```python
from build123d import *

# Parameters (mm, degrees)
BOSS_EXTRUDE1_DEPTH = 4
BOSS_EXTRUDE2_DEPTH = 8
BOSS_EXTRUDE3_DEPTH = 4
SKETCH4_R           = 2.6
CUT_EXTRUDE1_DEPTH  = 12
SKETCH5_W           = 20
SKETCH5_H           = 20
CUT_EXTRUDE2_DEPTH  = 12


with BuildPart() as part:
    # Sketch1 → Boss-Extrude1 (new body)
    with BuildSketch(Plane(origin=(0, 0, 0), x_dir=(1, 0, 0), z_dir=(0, 1, 0))):
        with BuildLine():
            Line((21.403642989, 12.918361615), (25.455844123, 16.970562748))
            ThreePointArc((25.455844123, 16.970562748), (25.455844123, 25.455844123), (16.970562748, 25.455844123))
            Line((16.970562748, 25.455844123), (12.918361615, 21.403642989))
            ThreePointArc((12.918361615, 21.403642989), (0, 25), (-12.918361615, 21.403642989))
            Line((-12.918361615, 21.403642989), (-16.970562748, 25.455844123))
            ThreePointArc((-16.970562748, 25.455844123), (-25.455844123, 25.455844123), (-25.455844123, 16.970562748))
            Line((-25.455844123, 16.970562748), (-21.403642989, 12.918361615))
            ThreePointArc((-21.403642989, 12.918361615), (-25, 0), (-21.403642989, -12.918361615))
            Line((-21.403642989, -12.918361615), (-25.455844123, -16.970562748))
            ThreePointArc((-25.455844123, -16.970562748), (-25.455844123, -25.455844123), (-16.970562748, -25.455844123))
            Line((-16.970562748, -25.455844123), (-12.918361615, -21.403642989))
            ThreePointArc((-12.918361615, -21.403642989), (0, -25), (12.918361615, -21.403642989))
            Line((12.918361615, -21.403642989), (16.970562748, -25.455844123))
            ThreePointArc((16.970562748, -25.455844123), (25.455844123, -25.455844123), (25.455844123, -16.970562748))
            Line((25.455844123, -16.970562748), (21.403642989, -12.918361615))
            ThreePointArc((21.403642989, -12.918361615), (25, 0), (21.403642989, 12.918361615))
        make_face()
    extrude(amount=BOSS_EXTRUDE1_DEPTH)

    # Sketch2 → Boss-Extrude2 (add)
    with BuildSketch(Plane(origin=(0, 4, 0), x_dir=(1, 0, 0), z_dir=(0, 1, 0))):
        with BuildLine():
            Line((-1, 25), (-1, 22.477766793))
            ThreePointArc((-1, 22.477766793), (-4.389532245, 22.067668809), (-7.677989416, 21.149432109))
            Line((-7.677989416, 21.149432109), (-8.643206277, 23.479671745))
            ThreePointArc((-8.643206277, 23.479671745), (-9.574736419, 23.115458518), (-10.490965342, 22.71430488))
            Line((-10.490965342, 22.71430488), (-9.525748481, 20.384065244))
            ThreePointArc((-9.525748481, 20.384065244), (-10.316353506, 19.995570768), (-11.091145538, 19.576426912))
            Line((-11.091145538, 19.576426912), (-16.970562748, 25.455844123))
            ThreePointArc((-16.970562748, 25.455844123), (-25.455844123, 25.455844123), (-25.455844123, 16.970562748))
            Line((-25.455844123, 16.970562748), (-19.576426912, 11.091145538))
            ThreePointArc((-19.576426912, 11.091145538), (-19.995570768, 10.316353506), (-20.384065244, 9.525748481))
            Line((-20.384065244, 9.525748481), (-22.71430488, 10.490965342))
            ThreePointArc((-22.71430488, 10.490965342), (-23.115458518, 9.574736419), (-23.479671745, 8.643206277))
            Line((-23.479671745, 8.643206277), (-21.149432109, 7.677989416))
            ThreePointArc((-21.149432109, 7.677989416), (-22.067668809, 4.389532245), (-22.477766793, 1))
            Line((-22.477766793, 1), (-25, 1))
            ThreePointArc((-25, 1), (-25.019992006, 0), (-25, -1))
            Line((-25, -1), (-22.477766793, -1))
            ThreePointArc((-22.477766793, -1), (-22.067668809, -4.389532245), (-21.149432109, -7.677989416))
            Line((-21.149432109, -7.677989416), (-23.479671745, -8.643206277))
            ThreePointArc((-23.479671745, -8.643206277), (-23.115458518, -9.574736419), (-22.71430488, -10.490965342))
            Line((-22.71430488, -10.490965342), (-20.384065244, -9.525748481))
            ThreePointArc((-20.384065244, -9.525748481), (-19.995570768, -10.316353506), (-19.576426912, -11.091145538))
            Line((-19.576426912, -11.091145538), (-25.455844123, -16.970562748))
            ThreePointArc((-25.455844123, -16.970562748), (-25.455844123, -25.455844123), (-16.970562748, -25.455844123))
            Line((-16.970562748, -25.455844123), (-11.091145538, -19.576426912))
            ThreePointArc((-11.091145538, -19.576426912), (-10.316353506, -19.995570768), (-9.525748481, -20.384065244))
            Line((-9.525748481, -20.384065244), (-10.490965342, -22.71430488))
            ThreePointArc((-10.490965342, -22.71430488), (-9.574736419, -23.115458518), (-8.643206277, -23.479671745))
            Line((-8.643206277, -23.479671745), (-7.677989416, -21.149432109))
            ThreePointArc((-7.677989416, -21.149432109), (-4.389532245, -22.067668809), (-1, -22.477766793))
            Line((-1, -22.477766793), (-1, -25))
            ThreePointArc((-1, -25), (0, -25.019992006), (1, -25))
            Line((1, -25), (1, -22.477766793))
            ThreePointArc((1, -22.477766793), (4.389532245, -22.067668809), (7.677989416, -21.149432109))
            Line((7.677989416, -21.149432109), (8.643206277, -23.479671745))
            ThreePointArc((8.643206277, -23.479671745), (9.574736419, -23.115458518), (10.490965342, -22.71430488))
            Line((10.490965342, -22.71430488), (9.525748481, -20.384065244))
            ThreePointArc((9.525748481, -20.384065244), (10.316353506, -19.995570768), (11.091145538, -19.576426912))
            Line((11.091145538, -19.576426912), (16.970562748, -25.455844123))
            ThreePointArc((16.970562748, -25.455844123), (25.455844123, -25.455844123), (25.455844123, -16.970562748))
            Line((25.455844123, -16.970562748), (19.576426912, -11.091145538))
            ThreePointArc((19.576426912, -11.091145538), (19.995570768, -10.316353506), (20.384065244, -9.525748481))
            Line((20.384065244, -9.525748481), (22.71430488, -10.490965342))
            ThreePointArc((22.71430488, -10.490965342), (23.115458518, -9.574736419), (23.479671745, -8.643206277))
            Line((23.479671745, -8.643206277), (21.149432109, -7.677989416))
            ThreePointArc((21.149432109, -7.677989416), (22.067668809, -4.389532245), (22.477766793, -1))
            Line((22.477766793, -1), (25, -1))
            ThreePointArc((25, -1), (25.019992006, 0), (25, 1))
            Line((25, 1), (22.477766793, 1))
            ThreePointArc((22.477766793, 1), (22.067668809, 4.389532245), (21.149432109, 7.677989416))
            Line((21.149432109, 7.677989416), (23.479671745, 8.643206277))
            ThreePointArc((23.479671745, 8.643206277), (23.115458518, 9.574736419), (22.71430488, 10.490965342))
            Line((22.71430488, 10.490965342), (20.384065244, 9.525748481))
            ThreePointArc((20.384065244, 9.525748481), (19.995570768, 10.316353506), (19.576426912, 11.091145538))
            Line((19.576426912, 11.091145538), (25.455844123, 16.970562748))
            ThreePointArc((25.455844123, 16.970562748), (25.455844123, 25.455844123), (16.970562748, 25.455844123))
            Line((16.970562748, 25.455844123), (11.091145538, 19.576426912))
            ThreePointArc((11.091145538, 19.576426912), (10.316353506, 19.995570768), (9.525748481, 20.384065244))
            Line((9.525748481, 20.384065244), (10.490965342, 22.71430488))
            ThreePointArc((10.490965342, 22.71430488), (9.574736419, 23.115458518), (8.643206277, 23.479671745))
            Line((8.643206277, 23.479671745), (7.677989416, 21.149432109))
            ThreePointArc((7.677989416, 21.149432109), (4.389532245, 22.067668809), (1, 22.477766793))
            Line((1, 22.477766793), (1, 25))
            ThreePointArc((1, 25), (0, 25.019992006), (-1, 25))
        make_face()
    extrude(amount=BOSS_EXTRUDE2_DEPTH)

    # Sketch3 → Boss-Extrude3 (add)
    with BuildSketch(Plane(origin=(0, 12, 0), x_dir=(1, 0, 0), z_dir=(0, 1, 0))):
        with BuildLine():
            Line((21.403642989, -12.918361615), (25.455844123, -16.970562748))
            ThreePointArc((25.455844123, -16.970562748), (25.455844123, -25.455844123), (16.970562748, -25.455844123))
            Line((16.970562748, -25.455844123), (12.918361615, -21.403642989))
            ThreePointArc((12.918361615, -21.403642989), (0, -25), (-12.918361615, -21.403642989))
            Line((-12.918361615, -21.403642989), (-16.970562748, -25.455844123))
            ThreePointArc((-16.970562748, -25.455844123), (-25.455844123, -25.455844123), (-25.455844123, -16.970562748))
            Line((-25.455844123, -16.970562748), (-21.403642989, -12.918361615))
            ThreePointArc((-21.403642989, -12.918361615), (-25, 0), (-21.403642989, 12.918361615))
            Line((-21.403642989, 12.918361615), (-25.455844123, 16.970562748))
            ThreePointArc((-25.455844123, 16.970562748), (-25.455844123, 25.455844123), (-16.970562748, 25.455844123))
            Line((-16.970562748, 25.455844123), (-12.918361615, 21.403642989))
            ThreePointArc((-12.918361615, 21.403642989), (0, 25), (12.918361615, 21.403642989))
            Line((12.918361615, 21.403642989), (16.970562748, 25.455844123))
            ThreePointArc((16.970562748, 25.455844123), (25.455844123, 25.455844123), (25.455844123, 16.970562748))
            Line((25.455844123, 16.970562748), (21.403642989, 12.918361615))
            ThreePointArc((21.403642989, 12.918361615), (25, 0), (21.403642989, -12.918361615))
        make_face()
    extrude(amount=BOSS_EXTRUDE3_DEPTH)

    # Sketch4 → Cut-Extrude1 (cut)
    with BuildSketch(Plane(origin=(0, 16, 0), x_dir=(1, 0, 0), z_dir=(0, 1, 0))):
        with Locations(Location((-21.213203436, -21.213203436, 0), (0, 0, 270))):
            Circle(SKETCH4_R)
        with Locations(Location((-21.213203436, 21.213203436, 0), (0, 0, 270))):
            Circle(SKETCH4_R)
        with Locations(Location((21.213203436, 21.213203436, 0), (0, 0, 270))):
            Circle(SKETCH4_R)
        with Locations(Location((21.213203436, -21.213203436, 0), (0, 0, 270))):
            Circle(SKETCH4_R)
    extrude(amount=-CUT_EXTRUDE1_DEPTH, mode=Mode.SUBTRACT)

    # Sketch5 → Cut-Extrude2 (cut)
    with BuildSketch(Plane(origin=(0, 16, 0), x_dir=(1, 0, 0), z_dir=(0, 1, 0))):
        Rectangle(SKETCH5_W, SKETCH5_H)
    extrude(amount=-CUT_EXTRUDE2_DEPTH, mode=Mode.SUBTRACT)


solid = part.part
```
Read the model definition and answer for the solid it produces. Units are mm, in the model's axes. A direction names the side the tool comes from. Give positions to 0.01 mm unless a question says otherwise; leave off trailing zeros. Order: outer loops, then holes, each group sorted by start corner. A loop starts at its lowest first (then second) coordinate and runs counter-clockwise, first axis right, second up. Notation, with made-up numbers: (-7, 0) -> (26, 0) arc R23 ccw to (26, 25) -> close; hole circle Ø11 at (67, 35.5). An arc over 180 degrees is marked (long way). Write item = value, one per line.
1. A cutting plane is placed at D-D, the plane y = 9. Count the separate pieces of the cut face and the enclosed holes in it, and give its area (3 significant figures).
Numbers:
separate_pieces = 1
enclosed_holes = 5
area = 1,770 mm²
2. A cutting plane is placed at B-B, the plane z = -3.5. Write down the section's boundary in (x, y).
Numbers:
outline = (-24.75, 0) -> (24.75, 0) -> (24.75, 4) -> (22.23, 4) -> (22.23, 12) -> (24.75, 12) -> (24.75, 16) -> (10, 16) -> (10, 4) -> (-10, 4) -> (-10, 16) -> (-24.75, 16) -> (-24.75, 12) -> (-22.23, 12) -> (-22.23, 4) -> (-24.75, 4) -> close
3. A cutting plane is placed at A-A, the plane y = 1. Write down the section's boundary in (x, z), and give its area (3 significant figures).
Numbers:
outline = (-25.46, -16.97) arc R6 ccw to (-16.97, -25.46) -> (-12.92, -21.4) arc R25 ccw to (12.92, -21.4) -> (16.97, -25.46) arc R6 ccw to (25.46, -16.97) -> (21.4, -12.92) arc R25 ccw to (21.4, 12.92) -> (25.46, 16.97) arc R6 ccw to (16.97, 25.46) -> (12.92, 21.4) arc R25 ccw to (-12.92, 21.4) -> (-16.97, 25.46) arc R6 ccw to (-25.46, 16.97) -> (-21.4, 12.92) arc R25 ccw to (-21.4, -12.92) -> close
area = 2,440 mm²
4. A cutting plane is placed at C-C, the plane x = 14. Write down the section's boundary in (y, z), and give its area (3 significant figures).
Numbers:
outline = (0, -22.49) -> (16, -22.49) -> (16, 22.49) -> (0, 22.49) -> close
area = 720 mm²
5. Given pin 1 (3 mm diameter, centred on x = -15, y = 8, fed in from -Z); pin 2 (1.5 mm diameter, centred on x = -1, z = -8, fed in from +Y); pin 3 (1 mm diameter, centred on x = 19.5, y = 2, fed in from +Z); pin 4 (0.6 mm diameter, centred on x = 10, z = -23.5, fed in from +Y), each flat-ended and moving along its own axis, determine where each tip first touches the part or whether it passes through.
Numbers:
pin_1 = -24.99
pin_2 = 4
pin_3 = 27.09
pin_4 = through
6. For faces 1 (the face through (-23.11, 7.94, -9.59)), 2 (the face through (-24, 8, 1)), 3 (the face through (10.015, 7.944, 21.565)), determine the directions among +Z, -Z, +X, -X, +Y, -Y from which every point of the face is accessible in a straight line to the end or side of a thin tool.
Numbers:
face_1 = -X, +Y, -Y
face_2 = -X
face_3 = none
7. Straight lines are drawn through the part: line 1 along Z through (x, y) = (20.5, 7); line 2 along Z through (x, y) = (22.5, 1.25); line 3 along Y through (x, z) = (8, -22). For each, find the intervals that lie inside material, in ascending order.
Numbers:
line_1 = -27.17 to -23.71, -18.71 to -12.01, -9.57 to 9.57, 12.01 to 18.71, 23.71 to 27.17
line_2 = -27.07 to -14.01, -10.9 to 10.9, 14.01 to 27.07
line_3 = 0 to 4, 12 to 16
8. The mould has two halves that part along Z. Classify faces 4 (the face through (0, 2, -25)), 5 (the face through (-0.01, 7.94, 25.02)), 6 (the face through (-11, 12, 21)): +Z half, -Z half, draft (parallel to the pull), parting line (faces both ways), or undercut.
Numbers:
face_4 = -Z half
face_5 = +Z half
face_6 = undercut
